Can you work these out from the model? Positions are in its coordinate system, mm. A direction names the side the tool comes from. Coordinates: 2 decimals unless noted, no trailing zeros. Order: outer loops, then holes, each group sorted by start corner. A loop starts at its lowest first (then second) coordinate and runs counter-clockwise, first axis right, second up. Notation, with made-up numbers: (44, -25.75) -> (85, -25.75) arc R17 ccw to (85, -6.75) -> close; hole circle Ø9 at (22, -19.5). An arc over 180 degrees is marked (long way). Answer in a Markdown table with one row per item.
```python
from build123d import *

# Parameters (mm, degrees)
SKETCH_1_R                  = 6.5
EXTRUDE_1_DEPTH             = 26
SKETCH_2_R                  = 2.85
CUT_EXTRUDE_1_DEPTH         = 3.5
HOLE_WIZARD_M32_D           = 3.4
HOLE_WIZARD_M32_CSINK_D     = 6.3
HOLE_WIZARD_M32_CSINK_ANGLE = 90


with BuildPart() as part:
    # Эскиз1 → Бобышка-Вытянуть1 (new body)
    with BuildSketch(Plane(origin=(0, 0, 0), x_dir=(1, 0, 0), z_dir=(0, 1, 0))):
        with Locations(Location((0, 0, 0), (0, 0, 90))):
            Circle(SKETCH_1_R)
    extrude(amount=EXTRUDE_1_DEPTH)

    # Эскиз2 → Вырез-Вытянуть1 (cut)
    with BuildSketch(Plane.XZ):
        with Locations(Location((0, 0, 0), (0, 0, 270))):
            Circle(SKETCH_2_R)
    extrude(amount=-CUT_EXTRUDE_1_DEPTH, mode=Mode.SUBTRACT)

    # Зенковка для  винта с плоской головкой M32 (through all)
    with Locations(Plane(origin=(0, 26, 0), x_dir=(1, 0, 0), z_dir=(0, 1, 0))):
        with Locations((0, 0)):
            CounterSinkHole(HOLE_WIZARD_M32_D / 2, HOLE_WIZARD_M32_CSINK_D / 2, counter_sink_angle=HOLE_WIZARD_M32_CSINK_ANGLE)


solid = part.part
```
(1) On a 3-axis mill with a long thin cutter (end or side, diameter ignored), from which of +Z, -Z, +X, -X, +Y, -Y can I reach the whole of each face in a straight line? I mean faces 1 (the flat face through (-2, 26, -3)), 2 (the cylindrical face through (-1.734, 1.726, 2.262)). Say none if no direction works.
Response values:
| item | result |
|---|---|
| face 1 | +Z, -Z, +X, -X, +Y |
| face 2 | -Y |
(2) Suppose I cut it at B-B (z = 0). Please give me the cut outline in (x, y), and give its area (3 significant figures).
Response values:
| item | result |
|---|---|
| outline | (-6.5, 0) -> (-2.85, 0) -> (-2.85, 3.5) -> (-1.7, 3.5) -> (-1.7, 24.55) -> (-3.15, 26) -> (-6.5, 26) -> close; (1.7, 3.5) -> (2.85, 3.5) -> (2.85, 0) -> (6.5, 0) -> (6.5, 26) -> (3.15, 26) -> (1.7, 24.55) -> close |
| area | 239 mm2 |
(3) Suppose I cut it at A-A (x = 0). Please give me the cut outline in (y, z).
Response values:
| item | result |
|---|---|
| outline | (0, -6.5) -> (26, -6.5) -> (26, -3.15) -> (24.55, -1.7) -> (3.5, -1.7) -> (3.5, -2.85) -> (0, -2.85) -> close; (0, 2.85) -> (3.5, 2.85) -> (3.5, 1.7) -> (24.55, 1.7) -> (26, 3.15) -> (26, 6.5) -> (0, 6.5) -> close |
(4) Will these pins go through, and if not, where does the flat tip stop? pin 1 Ø5 at (y, z) = (5.5, 3.5) entering from +X; pin 2 Ø5.5 at (x, z) = (0, 0) entering from +Y; pin 3 Ø1.7 at (x, z) = (-1, 0) entering from -Y.
Response values:
| item | result |
|---|---|
| pin 1 | x = 6.42 |
| pin 2 | y = 25.6 |
| pin 3 | y = 3.5 |
(5) Suppose I cut it at C-C (y = 8.5). Please give me the cut outline in (x, z), and give its area (3 significant figures).
Response values:
| item | result |
|---|---|
| outline | circle Ø13 at (0, 0); hole circle Ø3.4 at (0, 0) |
| area | 124 mm2 |
(6) I need wall thicknesses on line 1 (X direction, y = 2.35, z = 0); line 2 (X direction, y = 19, z = -1.25); line 3 (X direction, y = 17.5, z = 2.5). Which ranges of each line are inside material? Lowest first, please. Write a range as [from, to].
Response values:
| item | result |
|---|---|
| line 1 | [-6.5, -2.85], [2.85, 6.5] |
| line 2 | [-6.38, -1.15], [1.15, 6.38] |
| line 3 | [-6, 6] |
(7) We'd pull the mould along X, two halves only. Please class faces 3 (the cylindrical face through (3.955, 12.818, 5.158)), 4 (the cylindrical face through (0.37, 13.88, 1.66)), 5 (the flat face through (1, 0, -3)): +X half, -X half, draft (parallel to the pull), parting line (faces both ways), or undercut.
Response values:
| item | result |
|---|---|
| face 3 | parting line |
| face 4 | undercut |
| face 5 | draft |
(8) Suppose I cut it at D-D (z = 3.75). Please give me the cut outline in (x, y).
Response values:
| item | result |
|---|---|
| outline | (-5.31, 0) -> (5.31, 0) -> (5.31, 26) -> (-5.31, 26) -> close |
